The listing builds one solid part. Answer for the finished solid, in the listing's coordinates (mm). Give positions to 0.01 mm unless a question says otherwise; leave off trailing zeros. Write each loop counter-clockwise with the first axis right and the second up, starting at its lowest first coordinate (ties: lowest second). Pieces come first, ordered by that corner, then holes.
```python
from build123d import *

# Parameters (mm, degrees)
F1_DEPTH = 12.7
F2_W     = 12.7
F2_H     = 12.7
F3_DEPTH = 225.300032
F4_W     = 12.7
F4_H     = 25.4
F5_DEPTH = 12.7
F7_D     = 6.8
F7_DEPTH = 15.75
F7_TIP   = 2.0429261047
F9_D     = 5.1054
F9_DEPTH = 16.51
F9_TIP   = 1.5338169022


# Not quite as in the source:
# - a feature names something its author has since deleted; it is built from what else it names


with BuildPart() as f1:
    # F0 (on Front) → F1 (new body)
    with BuildSketch(Plane.XZ):
        Polygon((0, 25.4), (0, 0), (101.6, 0), (101.6, 226.6), (101.6, 239.3), (101.6, 252), (74.1228589826, 252), align=None)
        Polygon((78.5142949131, 226.6), (88.9, 226.6), (88.9, 12.7), (12.7, 12.7), (12.7, 25.4), align=None, mode=Mode.SUBTRACT)
    extrude(amount=F1_DEPTH)

    # F2 (on face) → F3 (join)
    with BuildSketch(Plane(origin=(0, 0, 0), x_dir=(-1, 0, 0), z_dir=(0, 1, 0))):
        with Locations((-95.25, 6.35)):
            Rectangle(F2_W, F2_H)
        Polygon((-101.6, 252), (-101.6, 226.6), (-88.9, 226.6), (-88.9, 229.1588783264), (-88.9, 252), align=None)
        Polygon((-12.7, 20.574), (-12.7, 12.7), (-12.7, 7.874), (0, 7.874), (0, 20.574), align=None)
    extrude(amount=F3_DEPTH)

    # F4 (on face) → F5 (join)
    with BuildSketch(Plane(origin=(0, 225.300032, 0), x_dir=(-1, 0, 0), z_dir=(0, 1, 0))):
        Polygon((0, 0), (0, 25.4), (-74.1228589826, 252), (-88.9, 252), (-88.9, 226.6), (-101.6, 226.6), (-101.6, 0), align=None)
        Polygon((-88.9, 25.4), (-88.9, 226.6), (-78.5142949131, 226.6), (-12.7, 25.4), (-12.7, 12.7), (-88.9, 12.7), align=None, mode=Mode.SUBTRACT)
        with Locations((-95.25, 239.3)):
            Rectangle(F4_W, F4_H)
    extrude(amount=F5_DEPTH)

    # F7
    with Locations(Plane.YZ.offset(101.6)):
        with Locations((-6.35, 19), (-6.35, 233), (231.650032, 233), (231.650032, 19)):
            Hole(F7_D / 2, depth=F7_DEPTH)
            with Locations((0, 0, -(F7_DEPTH + F7_TIP / 2))):  # 118° drill point
                Cone(0, F7_D / 2, F7_TIP, mode=Mode.SUBTRACT)

    # F9
    with Locations(Plane.XY.offset(252)):
        with Locations((95.25, 212.600032), (95.25, 12.7)):
            Hole(F9_D / 2, depth=F9_DEPTH)
            with Locations((0, 0, -(F9_DEPTH + F9_TIP / 2))):  # 118° drill point
                Cone(0, F9_D / 2, F9_TIP, mode=Mode.SUBTRACT)


solid = f1.part
```
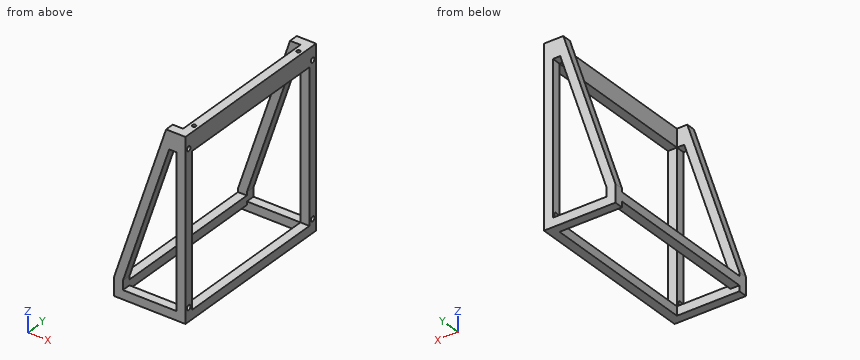
Item 1: A cutting plane is placed at A-A, the plane y = 171.5. Give the vertices of the cut face in (x, z), plus the area to 3 significant figures.
Conclusion:
outline: (0, 7.87) - (12.7, 7.87) - (12.7, 20.57) - (0, 20.57) - close; (88.9, 0) - (101.6, 0) - (101.6, 12.7) - (88.9, 12.7) - close; (88.9, 226.6) - (101.6, 226.6) - (101.6, 252) - (88.9, 252) - close
area: 645 mm2
Item 2: Consider probe 1 along Z at (x, y) = (96, -6); probe 2 along Y at (x, z) = (95, 244); probe 3 along Z at (x, y) = (96, 90). Determine where each line is inside the solid, lowest interval first.
Conclusion:
probe 1: z = 0 to 15.62, 22.38 to 229.62, 236.38 to 252
probe 2: y = -12.7 to 10.16, 15.24 to 210.06, 215.14 to 238
probe 3: z = 0 to 12.7, 226.6 to 252
Item 3: A cutting plane is placed at B-B, the plane z = 181.5. Give the vertices of the cut face in (x, y).
Conclusion:
outline: (51.06, -12.7) - (63.76, -12.7) - (63.76, 0) - (51.06, 0) - close; (51.06, 225.3) - (63.76, 225.3) - (63.76, 238) - (51.06, 238) - close; (88.9, -12.7) - (101.6, -12.7) - (101.6, 0) - (88.9, 0) - close; (88.9, 225.3) - (101.6, 225.3) - (101.6, 238) - (88.9, 238) - close
Item 4: Each of these flat-tipped pins is pushed along its axis until it touches: P1, Ø4, axis at y = -8, z = 113.5, coming from the -X side; P2, Ø14, axis at x = 9, y = 128.5, coming from the +Z side; P3, Ø4, axis at x = 4, y = 62, coming from the -Z side. Where does it stop, or does it pass through?
Conclusion:
P1: stops at x = 28.16
P2: stops at z = 20.57
P3: stops at z = 7.87
Item 5: A cutting plane is placed at C-C, the plane x = 70.5. Give the vertices of the cut face in (y, z), plus the area to 3 significant figures.
Conclusion:
outline: (-12.7, 0) - (0, 0) - (0, 12.7) - (-12.7, 12.7) - close; (-12.7, 202.1) - (0, 202.1) - (0, 240.92) - (-12.7, 240.92) - close; (225.3, 0) - (238, 0) - (238, 12.7) - (225.3, 12.7) - close; (225.3, 202.1) - (238, 202.1) - (238, 240.92) - (225.3, 240.92) - close
area: 1,310 mm2
